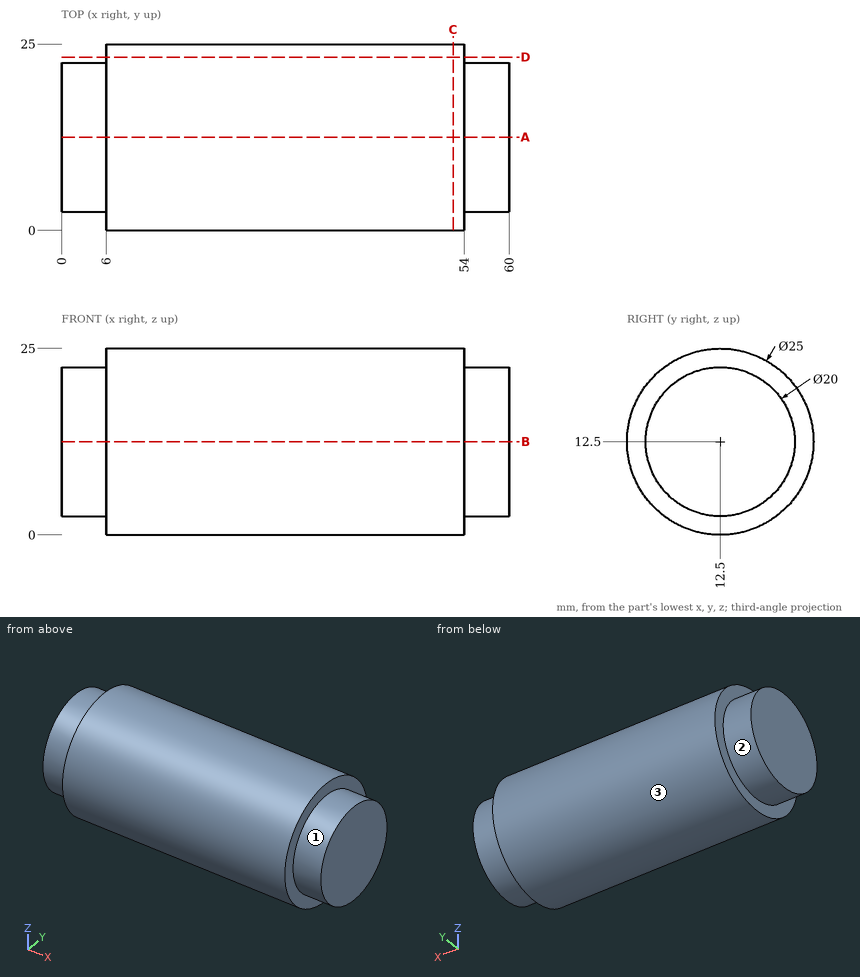
Print and shaded views of the part. All mm, measured from the part's lowest x, y and z. A direction names the side the tool comes from. Round coordinates to 2 decimals unless told otherwise and drop trailing zeros. Write each loop counter-clockwise with the first axis right and the second up, starting at its lowest first coordinate (ties: lowest second). Pieces come first, ordered by that corner, then holes. Notation, with made-up numbers: (62.5, -39) -> (92.5, -39) arc R15 cw to (92.5, -29) -> close; hole circle Ø3 at (5, 12.5). An arc over 180 degrees is marked (long way). Return JSON: item names as keys, results as strings. Group by question number.
Q1. Saw through at A-A on y = 12.5. Write the cut outline in (x, z).
Q2. Probe L1, parallel to X at y = 2.75, z = 18.5; L2, parallel to Z at x = 9, y = 12.5; L3, parallel to Y at x = 10.5, z = 13. List the from-to ranges inside material, lowest first. Write a range as [from, to].
Q3. Pin check, flat tips, straight feed: pin 1 (4 mm diameter, centred on x = 6.5, y = 21.5, fed in from -Z); pin 2 (1.5 mm diameter, centred on x = 29.5, z = 20, fed in from -Y); pin 3 (8 mm diameter, centred on x = 14, z = 4, fed in from +Y). Stop position of each tip, or through.
Q4. Which spindle directions (+Z, -Z, +X, -X, +Y, -Y) get a long thin tool onto all of the face, cutting with end or side? Do the marked faces 1, 2 and 3. Say none if no direction does.
Q5. Saw through at D-D on y = 23.25. Write the cut outline in (x, z).
Q6. Saw through at C-C on x = 52.5. Write the cut outline in (y, z).
Answer:
{
 "1": {"outline": "(0, 2.5) -> (6, 2.5) -> (6, 0) -> (54, 0) -> (54, 2.5) -> (60, 2.5) -> (60, 22.5) -> (54, 22.5) -> (54, 25) -> (6, 25) -> (6, 22.5) -> (0, 22.5) -> close"},
 "2": {"L1": "[6, 54]", "L2": "[0, 25]", "L3": "[0.01, 24.99]"},
 "3": {"pin 1": "z = 2.14", "pin 2": "y = 1.98", "pin 3": "y = 24.16"},
 "4": {"face 1": "+X", "face 2": "-X", "face 3": "+X, -X"},
 "5": {"outline": "(6, 6.12) -> (54, 6.12) -> (54, 18.88) -> (6, 18.88) -> close"},
 "6": {"outline": "circle Ø25 at (12.5, 12.5)"}
}
